Source: three-view drawing plus pictorial views. Frame: mm from the lowest corner of the part. A direction names the side the tool comes from. Give positions to 0.01 mm unless a question says otherwise; leave off trailing zeros. Write each loop counter-clockwise with the first axis right and the second up, starting at its lowest first coordinate (ties: lowest second). Pieces come first, ordered by that corner, then holes. Notation, with made-up numbers: M 66,-7 L 80,-7 A12 ccw 80,3 Z; hole C 73,72.5 d1. An arc over 180 degrees is marked long. One line per question, with ' | ' between items.
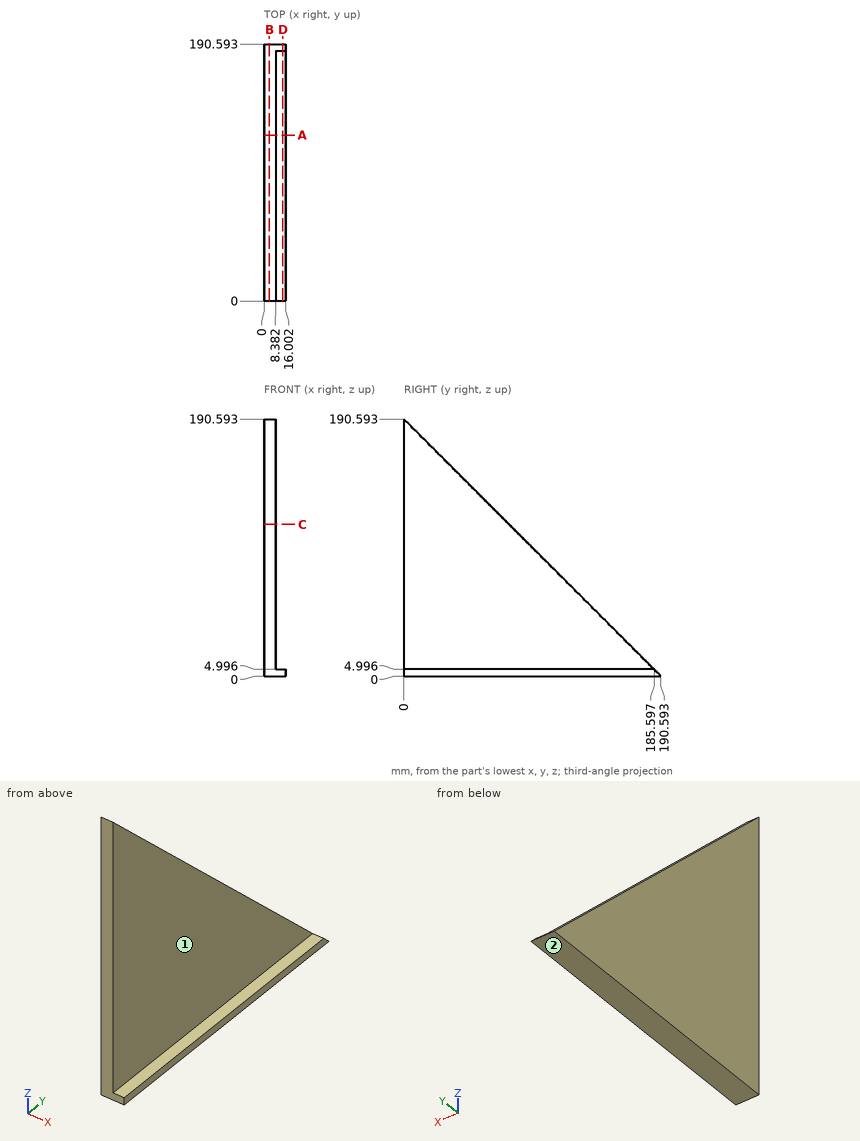
(1) Cut plane C-C, the plane z = 112.5. Return loops of the section in (x, y).
Working result:
outline: M 0,0 L 8.38,0 L 8.38,78.09 L 0,78.09 Z
(2) Material intervals for L1, parallel to X at y = 85.5, z = 32; L2, parallel to Z at x = 9.75, y = 46; L3, parallel to Y at x = 7.75, z = 52.5 (1 decimal), sorted ascending. Write a range as [from, to].
Working result:
L1: x = [0, 8.38] | L2: z = [0, 5] | L3: y = [0, 138.1]
(3) Cut plane B-B, the plane x = 3.75. Return loops of the section in (y, z).
Working result:
outline: M 0,0 L 190.59,0 L 0,190.59 Z
(4) First-contact query: P1, Ø6, axis at y = 118.5, z = 28.5, coming from the -X side; P2, Ø8, axis at x = 4.5, y = 97.5, coming from the +Z side (1 decimal); P3, Ø2.5, axis at x = 14, y = 74.5, coming from the +Z side; P4, Ø3, axis at x = 1.5, y = 34.5, coming from the +Z side (1 decimal). Flat tips, straight axial feed; report the tip coordinate or a pass-through.
Working result:
P1: stops at x = 0 | P2: stops at z = 97.1 | P3: stops at z = 5 | P4: stops at z = 157.6
(5) Cut plane A-A, the plane y = 123. Return loops of the section in (x, z).
Working result:
outline: M 0,0 L 16,0 L 16,5 L 8.38,5 L 8.38,67.59 L 0,67.59 Z
(6) Set-up query: the marked faces 1 and 2. Return all of +Z, -Z, +X, -X, +Y, -Y with unobstructed straight access to the full face (end or side cutting, diameter ignored); none if empty.
Working result:
face 1: +Z, +X, +Y, -Y | face 2: -Z, +X, -X, +Y, -Y
(7) Cut plane D-D, the plane x = 13.75. Return loops of the section in (y, z).
Working result:
outline: M 0,0 L 190.59,0 L 185.6,5 L 0,5 Z
